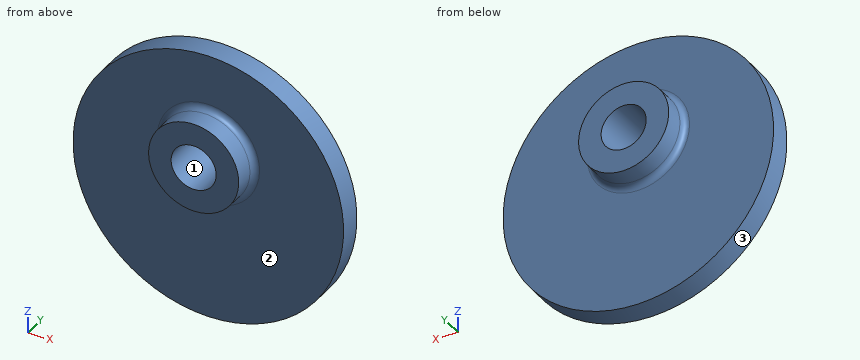
```python
from build123d import *

# Parameters (mm, degrees)
CROQUIS4_OUTSIDE_W    = 159.554
CROQUIS4_OUTSIDE_H    = 159.554
CROQUIS4_OUTSIDE_R    = 30
CORTAR_EXTRUIR9_DEPTH = 10


with BuildPart() as part:
    # Croquis1 → Revolución1 (revolve)
    with BuildSketch(Plane.XY, mode=Mode.PRIVATE) as revoluci_n1_sk:
        with BuildLine():
            Line((5, 8), (10, 8))
            Line((10, 8), (10.051225386, 3.891))
            ThreePointArc((10.051225386, 3.891), (10.39716845, 2.91351819), (11.348036475, 2.5))
            Line((11.348036475, 2.5), (61.351351351, 2.5))
            Line((61.351351351, 2.5), (61.351351351, -2.5))
            Line((61.351351351, -2.5), (11.351351351, -2.5))
            ThreePointArc((11.351351351, -2.5), (10.398380886, -2.912350032), (10.051351351, -3.891))
            Line((10.051351351, -3.891), (10, -8))
            Line((10, -8), (5, -8))
            Line((5, -8), (5, 8))
        make_face()
    revolve(revoluci_n1_sk.sketch.rotate(Axis((0, -587.784635029, 0), (0, 1, 0)), 90), axis=Axis((0, -587.784635029, 0), (0, 1, 0)))

    # Croquis4 outside → Cortar-Extruir9 (cut)
    with BuildSketch(Plane(origin=(0, 2.5, 0), x_dir=(1, 0, 0), z_dir=(0, 1, 0))):
        Rectangle(CROQUIS4_OUTSIDE_W, CROQUIS4_OUTSIDE_H)
        with Locations(Location((0, 7.5, 0), (0, 0, 270))):
            Circle(CROQUIS4_OUTSIDE_R, mode=Mode.SUBTRACT)
    extrude(amount=-CORTAR_EXTRUIR9_DEPTH, mode=Mode.SUBTRACT)


solid = part.part
```
Geometry: final body of the model. Coordinates: model frame, mm. Face numbers are marked on the shaded views. Round coordinates to 2 decimals unless told otherwise and drop trailing zeros. Order: outer loops, then holes, each group sorted by start corner. A loop starts at its lowest first (then second) coordinate and runs counter-clockwise, first axis right, second up. Notation, with made-up numbers: (23, 20) -> (75, 20) arc R27 ccw to (75, 46) -> close; hole circle Ø2 at (57.5, -37.75). An arc over 180 degrees is marked (long way). Use CSV: the item, a comma, the result in double quotes. Start each with the question number.
1) First-contact query: pin 1 Ø2 at (x, z) = (-12.5, -4) entering from -Y; pin 2 Ø1.5 at (x, y) = (11, -1) entering from -Z; pin 3 Ø4 at (x, y) = (10.5, 2) entering from +Z. Flat tips, straight axial feed; report the tip coordinate or a pass-through.
2) Material intervals for line 1 along X through (y, z) = (4.75, 0); line 2 along Y through (x, z) = (11.5, 0.5); line 3 along X through (y, z) = (-3.5, -2), sorted ascending. Write a range as from..to.
3) Draft query along Z for the marked faces 1, 2 and 3. Return one class per face: +Z half, -Z half, draft (parallel to the pull), parting line (faces both ways), or undercut.
4) Section B-B (x = 26). Return the cut outline in (y, z), and give its area (3 significant figures).
5) Section A-A (y = 6). Return the cut outline in (x, z).
6) Section C-C (z = 17). Return the cut outline in (x, y), and give its area (3 significant figures).
Returned:
1,pin 1,"stops at y = -2.5"
1,pin 2,"stops at z = -35.69"
1,pin 3,"stops at z = 21.27"
2,line 1,"x = -10.04..-5, 5..10.04"
2,line 2,"y = -2.5..2.5"
2,line 3,"x = -9.88..-4.58, 4.58..9.88"
3,face 1,"undercut"
3,face 2,"draft"
3,face 3,"parting line"
4,outline,"(-2.5, -22.47) -> (2.5, -22.47) -> (2.5, 7.47) -> (-2.5, 7.47) -> close"
4,area,"150 mm²"
5,outline,"circle Ø20.05 at (0, 0); hole circle Ø10 at (0, 0)"
6,outline,"(-17.31, -2.5) -> (17.31, -2.5) -> (17.31, 2.5) -> (-17.31, 2.5) -> close"
6,area,"173 mm²"
